from build123d import *

# Parameters (mm, degrees)
F1_DEPTH  = 39.766
F2_R      = 4.8
F3_DEPTH  = 39.767
F2_R_2    = 6.35
F4_DEPTH  = 1.5875
F5_R      = 6.35
F6_DEPTH  = 1.5875
F7_W      = 7.5
F7_H      = 19.36
F8_DEPTH  = 7.1
F10_DEPTH = 19.3
F11_R     = 2
F12_R     = 0.5


with BuildPart() as f1:
    # F0 (on Front) → F1 (new body)
    with BuildSketch(Plane.XZ):
        Polygon((0, 27.9), (0, 0), (37, 0), (37, 8.6), (14, 8.6), (14, 27.9), align=None)
    extrude(amount=F1_DEPTH)

    # F2 (on face) → F3 (cut, through all)
    with BuildSketch(Plane.XZ.offset(39.766)):
        with Locations((7, 17.55)):
            Circle(F2_R)
    extrude(amount=-F3_DEPTH, mode=Mode.SUBTRACT)

    # F2 (on face) → F4 (cut)
    with BuildSketch(Plane.XZ.offset(39.766)):
        with Locations((7, 17.55)):
            Circle(F2_R_2)
        with Locations((7, 17.55)):
            Circle(F2_R, mode=Mode.SUBTRACT)
    extrude(amount=-F4_DEPTH, mode=Mode.SUBTRACT)

    # F5 (on face) → F6 (cut)
    with BuildSketch(Plane.XZ):
        with Locations((7, 17.55)):
            Circle(F5_R)
    extrude(amount=F6_DEPTH, mode=Mode.SUBTRACT)

    # F7 (on face) → F8 (cut)
    with BuildSketch(Plane.XY.offset(8.6)):
        with Locations((10.25, -19.883)):
            Rectangle(F7_W, F7_H)
        Polygon((37, -28.563), (37, -11.203), (35, -11.203), (35, -10.203), (14, -10.203), (14, -29.563), (35, -29.563), (35, -28.563), align=None)
    extrude(amount=-F8_DEPTH, mode=Mode.SUBTRACT)

    # F9 (on face) → F10 (cut, through all)
    with BuildSketch(Plane.XY.offset(27.9)):
        Polygon((0, -12.827), (0, -19.883), (0, -26.939), (14, -26.939), (14, -12.827), align=None)
    extrude(amount=-F10_DEPTH, mode=Mode.SUBTRACT)

    # F11
    f11_edges = [f1.edges().sort_by_distance(p)[0] for p in [
        (10.25, -26.939, 8.6),
        (14, -11.515, 8.6),
        (10.25, -12.827, 8.6),
        (14, -28.251, 8.6),
    ]]
    fillet(f11_edges, radius=F11_R)

    # F12
    f12_edges = [f1.edges().sort_by_distance(p)[0] for p in [
        (24.5, -10.203, 8.6),
        (24.5, -29.563, 8.6),
        (6.5, -19.883, 8.6),
        (37, -5.6015, 8.6),
        (37, -34.1645, 8.6),
        (37, -28.563, 5.05),
        (35, -11.203, 5.05),
        (37, -19.883, 1.5),
        (35, -29.063, 8.6),
        (35, -28.563, 5.05),
        (36, -28.563, 8.6),
        (36, -11.203, 8.6),
        (35, -10.703, 8.6),
        (25.5, 0, 8.6),
        (25.5, -39.766, 8.6),
        (14, -33.3525, 27.9),
        (7, -26.939, 27.9),
        (0, -33.3525, 27.9),
        (7, -39.766, 27.9),
        (7, -12.827, 27.9),
        (0, -19.883, 8.6),
        (0, -6.4135, 27.9),
        (7, 0, 27.9),
        (14, -6.4135, 27.9),
        (14, -12.827, 19.25),
        (0, -12.827, 18.25),
        (0, 0, 13.95),
        (0, -19.883, 0),
        (0, -39.766, 13.95),
        (14, -39.766, 18.25),
        (14, -26.939, 19.25),
        (14, 0, 18.25),
        (18.5, -39.766, 0),
        (37, -19.883, 0),
        (37, -39.766, 4.3),
        (37, 0, 4.3),
        (0, -26.939, 18.25),
        (13.414214, -12.241214, 9.185786),
        (13.414214, -27.524786, 9.185786),
    ]]
    fillet(f12_edges, radius=F12_R)


solid = f1.part
Here's how the part is built. I have some questions about the finished solid (model axes, mm). A direction names the side the tool comes from. Give positions to 0.01 mm unless a question says otherwise; leave off trailing zeros. Loops run counter-clockwise (first coordinate to the right, second up) from the corner with the lowest first, then second, coordinate; pieces in that order, holes last. Notation, with made-up numbers: (76, 30.25) -> (129, 30.25) arc R22 cw to (129, 69.25) -> close; hole circle Ø6 at (51.25, 14.5). An arc over 180 degrees is marked (long way). Answer as a JSON object with one key per item and string values. Group by question number.
Item 1: Thinking about a two-plate mould opening in Z: for faces 1 (the flat face through (7, -6, 27.9)), 2 (the flat face through (37, -11, 4)), 3 (the cylindrical face through (11.434, -32.637, 15.712)), which applies, pulls with the +Z half, pulls with the -Z half, needs draft (parallel to the pull), parting line crosses it, or undercut?
Item 2: On a 3-axis mill with a long thin cutter (end or side, diameter ignored), from which of +Z, -Z, +X, -X, +Y, -Y can I reach the whole of each face in a straight line? I mean faces 4 (the flat face through (25, -4, 8.6)), 5 (the flat face through (3, -20, 8.6)), 6 (the flat face through (5.6, -1.588, 22.3)). Say none if no direction works.
Item 3: Imagine slicing it at C-C on x = 24.5. Write out the boundary of the cut face in (y, z).
Item 4: Will these pins go through, and if not, where does the flat tip stop? pin 1 (7.5 mm diameter, centred on x = 7, z = 17.55, fed in from +Y); pin 2 (3.5 mm diameter, centred on y = -35.5, z = 15.5, fed in from +X); pin 3 (4 mm diameter, centred on x = 5.5, z = 14, fed in from -Y); pin 4 (7.5 mm diameter, centred on y = -19, z = 5.5, fed in from +X).
Item 5: I need wall thicknesses on L1, parallel to Z at x = 7, y = -29.5; L2, parallel to Y at x = 8, z = 23.5; L3, parallel to X at y = -3, z = 17.5. Which ranges of each line are inside material? Lowest first, please.
Item 6: Imagine slicing it at A-A on z = 21. Give the number of separate pieces and of enclosed holes in the cut face, then the cut area to 3 significant figures.
Item 7: Imagine slicing it at D-D on y = -13.5. Write out the boundary of the cut face in (x, z), then the cut area to 3 significant figures.
Item 8: Imagine slicing it at B-B on y = -3.5. Write out the boundary of the cut face in (x, z), then the cut area to 3 significant figures.
Answer list:
{
 "1": {"face 1": "pulls with the +Z half", "face 2": "needs draft", "face 3": "undercut"},
 "2": {"face 4": "+Z, +X, +Y, -Y", "face 5": "+Z, +X, -X", "face 6": "+Y"},
 "3": {"outline": "(-39.77, 0.5) arc R0.5 ccw to (-39.27, 0) -> (0, 0) -> (0, 8.1) arc R0.5 ccw to (-0.5, 8.6) -> (-9.7, 8.6) arc R0.5 ccw to (-10.2, 8.1) -> (-10.2, 1.5) -> (-29.56, 1.5) -> (-29.56, 8.1) arc R0.5 ccw to (-30.06, 8.6) -> (-39.27, 8.6) arc R0.5 ccw to (-39.77, 8.1) -> close"},
 "4": {"pin 1": "passes through", "pin 2": "stops at x = 14", "pin 3": "stops at y = -38.18", "pin 4": "stops at x = 6.5"},
 "5": {"L1": "z = 0 to 1.5, 8.6 to 12.75, 22.35 to 27.9", "L2": "y = -38.18 to -26.94, -12.83 to -1.59", "L3": "x = 0 to 2.2, 11.8 to 14"},
 "6": {"separate pieces": "4", "enclosed holes": "0", "area": "175 mm2"},
 "7": {"outline": "(0, 0.5) arc R0.5 ccw to (0.5, 0) -> (36.5, 0) arc R0.5 ccw to (37, 0.5) -> (37, 1) arc R0.5 ccw to (36.5, 1.5) -> (6.5, 1.5) -> (6.5, 8.1) arc R0.5 ccw to (6, 8.6) -> (0.5, 8.6) arc R0.5 ccw to (0, 8.1) -> close", "area": "101 mm2"},
 "8": {"outline": "(0, 0.5) arc R0.5 ccw to (0.5, 0) -> (36.5, 0) arc R0.5 ccw to (37, 0.5) -> (37, 8.1) arc R0.5 ccw to (36.5, 8.6) -> (14, 8.6) -> (14, 27.4) arc R0.5 ccw to (13.5, 27.9) -> (0.5, 27.9) arc R0.5 ccw to (0, 27.4) -> close; hole circle Ø9.6 at (7, 17.55)", "area": "516 mm2"}
}
